Verification items for the finished model (mm, model axes). Face numbers are marked on the shaded views. A direction names the side the tool comes from. Round coordinates to 2 decimals unless told otherwise and drop trailing zeros. Write each loop counter-clockwise with the first axis right and the second up, starting at its lowest first coordinate (ties: lowest second). Pieces come first, ordered by that corner, then holes. Notation, with made-up numbers: (74, -31.5) - (116, -31.5) arc R20 cw to (116, -24.5) - close; hole circle Ø8 at (5, -4.5). An arc over 180 degrees is marked (long way). Answer as a JSON object with one key per item and string values.
```python
from build123d import *

# Parameters (mm, degrees)
SKETCH1_R          = 14.2875
EXTRUDE1_DEPTH     = 4.318
SKETCH2_R          = 16.002
EXTRUDE2_DEPTH     = 8.255
SKETCH3_R          = 16.383
EXTRUDE3_DEPTH     = 7.62
SKETCH4_R          = 16.002
EXTRUDE4_DEPTH     = 23.368
SKETCH5_R          = 15.24
CUT_EXTRUDE1_DEPTH = 1.27
SKETCH6_R          = 10.16
CUT_EXTRUDE2_DEPTH = 5.08


with BuildPart() as part:
    # Sketch1 → Extrude1 (new body)
    with BuildSketch(Plane.XY):
        Circle(SKETCH1_R)
    extrude(amount=EXTRUDE1_DEPTH)

    # Sketch2 → Extrude2 (add)
    with BuildSketch(Plane.XY.offset(4.318)):
        Circle(SKETCH2_R)
    extrude(amount=EXTRUDE2_DEPTH)

    # Sketch3 → Extrude3 (add)
    with BuildSketch(Plane.XY.offset(12.573)):
        Circle(SKETCH3_R)
    extrude(amount=EXTRUDE3_DEPTH)

    # Sketch4 → Extrude4 (add)
    with BuildSketch(Plane.XY.offset(20.193)):
        Circle(SKETCH4_R)
    extrude(amount=EXTRUDE4_DEPTH)

    # Sketch5 → Cut-Extrude1 (cut)
    with BuildSketch(Plane.XY.offset(43.561)):
        Circle(SKETCH5_R)
    extrude(amount=-CUT_EXTRUDE1_DEPTH, mode=Mode.SUBTRACT)

    # Sketch6 → Cut-Extrude2 (cut)
    with BuildSketch(Plane.XY.offset(42.291)):
        Circle(SKETCH6_R)
    extrude(amount=-CUT_EXTRUDE2_DEPTH, mode=Mode.SUBTRACT)


solid = part.part
```
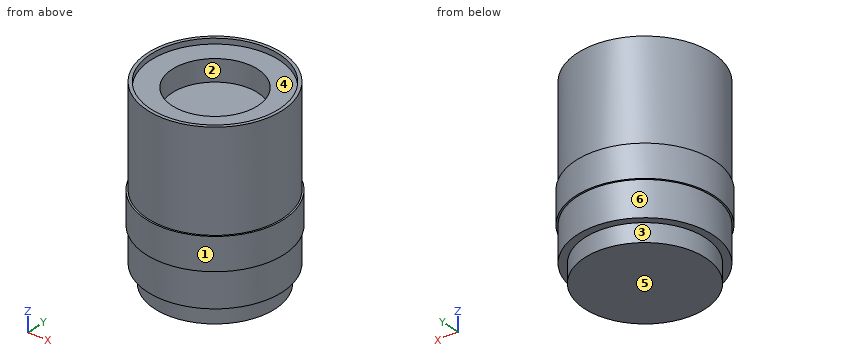
Q1. Section check C-C, the plane z = 40. Record the cut outline in (x, y).
Geometry check:
{"outline": "circle Ø32 at (0, 0); hole circle Ø20.32 at (0, 0)"}
Q2. Gauge pin test, flat ends, axial feed: P1, Ø1, axis at y = -7, z = 23.5, coming from the -X side; P2, Ø16.5, axis at x = 1, y = 3.5, coming from the +Z side; P3, Ø1, axis at x = -4.5, z = 9, coming from the -Y side. Record the tip position at first contact, or that the pin passes through.
Geometry check:
{"P1": "stops at x = -14.62", "P2": "stops at z = 42.29", "P3": "stops at y = -15.49"}
Q3. Section check D-D, the plane z = 32.5. Record the cut outline in (x, y), then the cut area to 3 significant figures.
Geometry check:
{"outline": "circle Ø32 at (0, 0)", "area": "804 mm2"}
Q4. Release check for a two-part mould opening along X. For the marked faces 4, 5 and 6 record: released by +X, released by -X, zero draft, split by the parting line, or undercut.
Geometry check:
{"face 4": "undercut", "face 5": "zero draft", "face 6": "split by the parting line"}
Q5. Material ranges on line 1 along Y through (x, z) = (0, 42.85); line 2 along Y through (x, z) = (0, 40.45); line 3 along X through (y, z) = (8, 40), recorded low to high. Write a range as [from, to].
Geometry check:
{"line 1": "y = [-16, -15.24], [15.24, 16]", "line 2": "y = [-16, -10.16], [10.16, 16]", "line 3": "x = [-13.86, -6.26], [6.26, 13.86]"}
Q6. Section check A-A, the plane x = 0. Record the cut outline in (y, z), then the cut area to 3 significant figures.
Geometry check:
{"outline": "(-16.38, 12.57) - (-16, 12.57) - (-16, 4.32) - (-14.29, 4.32) - (-14.29, 0) - (14.29, 0) - (14.29, 4.32) - (16, 4.32) - (16, 12.57) - (16.38, 12.57) - (16.38, 20.19) - (16, 20.19) - (16, 43.56) - (15.24, 43.56) - (15.24, 42.29) - (10.16, 42.29) - (10.16, 37.21) - (-10.16, 37.21) - (-10.16, 42.29) - (-15.24, 42.29) - (-15.24, 43.56) - (-16, 43.56) - (-16, 20.19) - (-16.38, 20.19) - close", "area": "1,240 mm2"}
Q7. Set-up check for the marked faces 1, 2 and 3: record each of +Z, -Z, +X, -X, +Y, -Y from which the full face is reachable in a straight line by a thin tool's end or side.
Geometry check:
{"face 1": "+Z, -Z", "face 2": "+Z", "face 3": "-Z"}
